Here's how the part is built. I have some questions about the finished solid (model axes, mm). Face numbers are marked on the shaded views. A direction names the side the tool comes from. Coordinates: 2 decimals unless noted, no trailing zeros. Write each loop counter-clockwise with the first axis right and the second up, starting at its lowest first coordinate (ties: lowest second). Pieces come first, ordered by that corner, then holes. Notation, with made-up numbers: M -17,-20 L 26,-20 A31 ccw 26,13 Z; hole C 8.5,75 d11. An arc over 180 degrees is marked long. Use one line per item in the form item = value. Start each with the question number.
1. I want a section at B-B, the plane z = -6. List the corners of the cut face in (x, y) for me.
2. On a 3-axis mill with a long thin cutter (end or side, diameter ignored), from which of +Z, -Z, +X, -X, +Y, -Y can I reach the whole of each face in a straight line? I mean the marked faces 4, 5, 6 and 7. Say none if no direction works.
3. Please list where these lines run through material, in increasing order: line 1 along Z through (x, y) = (-1, 6.25); line 2 along Y through (x, z) = (-4.75, -22); line 3 along Z through (x, y) = (-4, 16). Write a range as [from, to].
4. I want a section at C-C, the plane x = 1.75. Count the separate pieces of the cut face and the enclosed holes in it, plus the area to 3 significant figures.
5. I want a section at D-D, the plane y = 14.75. List the corners of the cut face in (x, z) for me.
6. I'm going to push flat-ended pins straight in: pin 1 Ø5 at (x, y) = (-3, 10.5) entering from +Z; pin 2 Ø6.5 at (x, z) = (0.5, 19.5) entering from -Y; pin 3 Ø10 at (x, y) = (0, 12.5) entering from -Z; pin 4 Ø1 at (y, z) = (6.5, 13.5) entering from +X. Where does each tip first touch, or does it pass through?
7. I want a section at A-A, the plane y = 6.25. List the corners of the cut face in (x, z) for me.
8. Thinking about a two-plate mould opening in Y: for the marked faces 1, 2 and 3, which applies, released by +Y, released by -Y, zero draft, split by the parting line, or undercut?
Autodesk Inventor part; units mm, degrees
ref_plane "YZ Plane" through (0, 0, 0) normal (1, 0, 0) x (0, 1, 0)
ref_plane "XZ Plane" through (0, 0, 0) normal (0, 1, 0) x (-1, 0, 0)
ref_plane "XY Plane" through (0, 0, 0) normal (0, 0, 1) x (1, 0, 0)
sketch "Sketch1" plane through (0, 0, 0) normal (0, 1, 0) x (-1, 0, 0)
  line L0 (5.25, 27.1768) -> (-5.25, 27.1768)
  line L1 (-5.25, 27.1768) -> (-9, 19.3232)
  line L2 (-9, 19.3232) -> (-9, -19.3232)
  line L3 (-9, -19.3232) -> (-5.25, -27.1768)
  line L4 (-5.25, -27.1768) -> (5.25, -27.1768)
  line L5 (5.25, -27.1768) -> (9, -19.3232)
  line L6 (9, -19.3232) -> (9, 19.3232)
  line L7 (9, 19.3232) -> (5.25, 27.1768)
  line L8 (4.25, 25.6768) -> (-4.25, 25.6768)
  line L9 (-4.25, 25.6768) -> (-4.25, 19.3232)
  line L10 (-4.25, 19.3232) -> (4.25, 19.3232)
  line L11 (4.25, 19.3232) -> (4.25, 25.6768)
  line L12 (4.25, -19.3232) -> (-4.25, -19.3232)
  line L13 (-4.25, -19.3232) -> (-4.25, -25.6768)
  line L14 (-4.25, -25.6768) -> (4.25, -25.6768)
  line L15 (4.25, -25.6768) -> (4.25, -19.3232)
  point P0 (0, 0)
  point P1 (0, 22.5)
  point P2 (0, -22.5)
  point P3 (0, 25.6768)
  point P4 (0, 27.1768)
  point P5 (0, -25.6768)
  point P6 (0, -27.1768)
  point P7 (4.25, 22.5)
  point P8 (0, 19.3232)
  point P9 (0, -19.3232)
  point P10 (4.25, -22.5)
  point P11 (9, 0)
  dimension "d0" = 18
  dimension "d1" = 1.5
  dimension "d2" = 1.5
  dimension "d3" = 8.5
  dimension "d4" = 8.5
  dimension "d6" = 10.5
  dimension "d7" = 10.5
  dimension "d8" = 9
  dimension "d12" = 115.524
  dimension "d13" = 115.524
  dimension "d14" = 115.524
  dimension "d15" = 115.524
  dimension "d16" = 45
extrude "Extrusion1" add sketch "Sketch1" along normal blind 3 contours L7 L6 L5 L4 L3 L2 L1 L0 | L11 L10 L9 L8 | L15 L14 L13 L12
sketch "Sketch2" plane through (0, 3, 0) normal (0, 1, 0) x (1, 0, 0)
  line L0 (5.25, -27.1768) -> (9, -19.3232)
  line L1 (9, -19.3232) -> (9, 19.3232)
  line L2 (9, 19.3232) -> (5.25, 27.1768)
  line L3 (5.25, 27.1768) -> (-5.25, 27.1768)
  line L4 (-5.25, 27.1768) -> (-9, 19.3232)
  line L5 (-9, 19.3232) -> (-9, -19.3232)
  line L6 (-9, -19.3232) -> (-5.25, -27.1768)
  line L7 (-5.25, -27.1768) -> (5.25, -27.1768)
  line L8 (-4.25, -25.6768) -> (4.25, -25.6768)
  line L9 (4.25, -25.6768) -> (4.25, -15.6768)
  line L10 (4.25, -15.6768) -> (-4.25, -15.6768)
  line L11 (-4.25, -15.6768) -> (-4.25, -25.6768)
  line L12 (-4.25, 15.6768) -> (4.25, 15.6768)
  line L13 (4.25, 15.6768) -> (4.25, 25.6768)
  line L14 (4.25, 25.6768) -> (-4.25, 25.6768)
  line L15 (-4.25, 25.6768) -> (-4.25, 15.6768)
  point P0 (0, 0)
  point P1 (0, -25.6768)
  point P2 (0, -27.1768)
  dimension "d19" = 1.5
  dimension "d20" = 1.5
  dimension "d21" = 8.5
  dimension "d22" = 8.5
  dimension "d23" = 10
  dimension "d24" = 10
extrude "Extrusion2" add sketch "Sketch2" along normal blind 15 contours L11 L10 L9 L8 | L15 L14 L13 L12
fillet "Fillet1" radius 5 4 edges at (0, 18, 25.6768) (0, 18, 15.6768) (0, 18, -15.6768) (0, 18, -25.6768)
sketch "Sketch3" plane through (4.25, 3, 25.6768) normal (1, 0, 0) x (0, 0, -1)
  arc A0 (10, 10) -> (0, 10) centre (5, 10) ccw
  line L0 (0, 0) -> (0, 10)
  line L1 (10, 0) -> (0, 0)
  line L2 (10, 0) -> (10, 10)
  circle A1 centre (5, 10) radius 1
  arc A2 (10, 10) -> (0, 10) centre (5, 10) ccw
  line L3 (2.4906, 14.3247) -> (1.0669, 16.8692)
  line L4 (1.0669, 16.8692) -> (0, 16.2723)
  line L5 (0, 16.2723) -> (1.5075, 13.5781)
  arc A3 (2.4906, 14.3247) -> (1.5075, 13.5781) centre (5, 10) ccw
  point P0 (25.6768, -3)
  point P1 (1.5075, 13.5781)
  point P2 (2.4906, 14.3247)
  dimension "d28" = 2
extrude "Extrusion3" add sketch "Sketch3" against normal up to surface (8.5 mm away) contours A0 L5 L4 L3
extrude "Extrusion4" cut sketch "Sketch3" against normal up to surface (8.5 mm away) contours A1
sketch "Sketch4" plane through (0, 3, 0) normal (0, 1, 0) x (1, 0, 0)
  line L0 (4.25, 15.6768) -> (-4.25, 15.6768)
  line L1 (-4.25, 15.6768) -> (-4.25, 25.6768)
  line L2 (-4.25, 25.6768) -> (4.25, 25.6768)
  line L3 (4.25, 25.6768) -> (4.25, 15.6768)
  line L4 (4.25, -25.6768) -> (-4.25, -25.6768)
  line L5 (-4.25, -25.6768) -> (-4.25, -15.6768)
  line L6 (-4.25, -15.6768) -> (4.25, -15.6768)
  line L7 (4.25, -15.6768) -> (4.25, -25.6768)
  line L8 (5.25, -27.1768) -> (9, -19.3232)
  line L9 (9, -19.3232) -> (9, 19.3232)
  line L10 (9, 19.3232) -> (5.25, 27.1768)
  line L11 (5.25, 27.1768) -> (-5.25, 27.1768)
  line L12 (-5.25, 27.1768) -> (-9, 19.3232)
  line L13 (-9, 19.3232) -> (-9, -19.3232)
  line L14 (-9, -19.3232) -> (-5.25, -27.1768)
  line L15 (-5.25, -27.1768) -> (5.25, -27.1768)
  line L16 (-7.5, 15.6768) -> (7.5, 15.6768)
  line L17 (7.5, 15.6768) -> (7.5, -15.6768)
  line L18 (7.5, -15.6768) -> (-7.5, -15.6768)
  line L19 (-7.5, -15.6768) -> (-7.5, 15.6768)
  point P0 (0, 0)
  dimension "d33" = 1.5
  dimension "d34" = 1.5
extrude "Extrusion5" cut sketch "Sketch4" against normal up to surface (3 mm away) contours L16 L17 L18 L6 L19 L0
sketch "Sketch5" plane through (4.25, 3, 25.6768) normal (1, 0, 0) x (0, 0, -1)
  line L0 (6.3537, 0) -> (45, 0)
  line L1 (2, 7) -> (8, 7)
  line L2 (8, 7) -> (8, 0)
  line L3 (8, 0) -> (2, 0)
  line L4 (2, 0) -> (2, 7)
  line L5 (0, 0) -> (0, 10)
  line L6 (10, 0) -> (10, 10)
  circle A0 centre (5, 10) radius 1
  point P0 (25.6768, -3)
  point P1 (6.3537, 0)
  dimension "d37" = 2
  dimension "d38" = 2
  dimension "d39" = 2
extrude "Extrusion6" cut sketch "Sketch5" against normal up to surface (8.5 mm away) contours L3 L4 L1 L2 L0
mirror "Mirror1" about plane through (0, 0, 0) normal (0, 0, 1) of "Extrusion3", "Extrusion6", "Extrusion4"
equation "\"d7\" = d6"
equation "\"d13\" = d12"
equation "\"d14\" = d12"
equation "\"d15\" = d12"
equation "\"d20\" = d19"
equation "\"d24\" = d23"
properties part number "PalmWithBackstop"
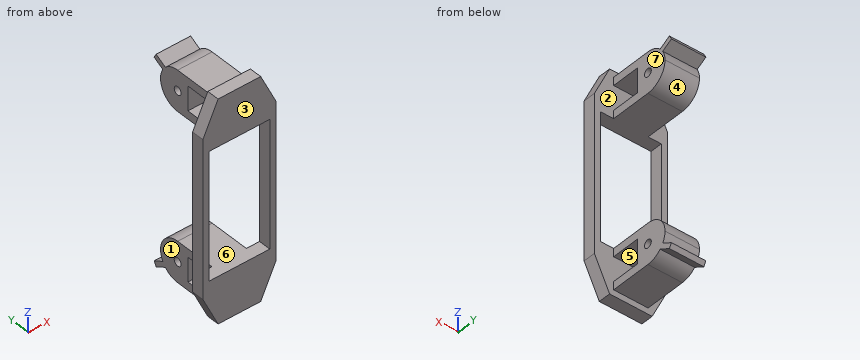
Answer list:
q1.outline = M -9,0 L -7.5,0 L -7.5,3 L -9,3 Z; M 7.5,0 L 9,0 L 9,3 L 7.5,3 Z
q2.face_4 = +X, -X, +Y
q2.face_5 = +X, -X
q2.face_6 = +Y, -Y
q2.face_7 = +Z, -Z, +X, +Y
q3.line_1 = [-25.68, -23.68], [-17.68, -15.68], [15.68, 17.68], [23.68, 25.68]
q3.line_2 = [0, 3]
q3.line_3 = [-24.68, -16.68], [16.68, 24.68]
q4.separate_pieces = 2
q4.enclosed_holes = 4
q4.area = 265 mm²
q5.outline = M -4.25,-25.36 L 4.25,-25.36 L 4.25,-15.99 L -4.25,-15.99 Z; M -4.25,15.99 L 4.25,15.99 L 4.25,25.36 L -4.25,25.36 Z
q6.pin_1 = 25.68
q6.pin_2 = 0
q6.pin_3 = -25.68
q6.pin_4 = through
q7.outline = M -4.25,-25.68 L 4.25,-25.68 L 4.25,-23.68 L -4.25,-23.68 Z; M -4.25,-17.68 L 4.25,-17.68 L 4.25,-15.68 L -4.25,-15.68 Z; M -4.25,15.68 L 4.25,15.68 L 4.25,17.68 L -4.25,17.68 Z; M -4.25,23.68 L 4.25,23.68 L 4.25,25.68 L -4.25,25.68 Z
q8.face_1 = zero draft
q8.face_2 = undercut
q8.face_3 = released by -Y
